from build123d import *

# Parameters (mm, degrees)
SKETCH1_W           = 94
SKETCH1_H           = 90
BOSS_EXTRUDE1_DEPTH = 12
SKETCH2_R           = 4
CUT_EXTRUDE1_DEPTH  = 67.166456759
SKETCH3_R           = 1.6
CUT_EXTRUDE2_DEPTH  = 67.166456759


with BuildPart() as part:
    # Sketch1 → Boss-Extrude1 (new body)
    with BuildSketch(Plane(origin=(0, 0, 0), x_dir=(0, 0, -1), z_dir=(1, 0, 0))):
        Rectangle(SKETCH1_W, SKETCH1_H)
    extrude(amount=BOSS_EXTRUDE1_DEPTH)

    # Sketch2 → Cut-Extrude1 (cut, through all)
    with BuildSketch(Plane(origin=(12, 0, 0), x_dir=(0, 0, -1), z_dir=(1, 0, 0))):
        Circle(SKETCH2_R)
    extrude(amount=-CUT_EXTRUDE1_DEPTH, mode=Mode.SUBTRACT)

    # Sketch3 → Cut-Extrude2 (cut, through all)
    with BuildSketch(Plane.ZY):
        with Locations((0, -20)):
            Circle(SKETCH3_R)
    extrude(amount=-CUT_EXTRUDE2_DEPTH, mode=Mode.SUBTRACT)


solid = part.part
Geometry: final body of the model. Coordinates: model frame, mm. Coordinates: 2 decimals unless noted, no trailing zeros. Loops run counter-clockwise (first coordinate to the right, second up) from the corner with the lowest first, then second, coordinate; pieces in that order, holes last. Notation, with made-up numbers: (41.25, 71) - (75.25, 71) arc R5 ccw to (75.25, 77) - close; hole circle Ø1 at (25.5, 71). An arc over 180 degrees is marked (long way). Put each result on its own line as item: value. Start each with the question number.
Q1. Line query: line 1 (Y direction, x = 4.5, z = 0). Output: solid intervals per line, ascending.
Q2. Cut plane A-A, the plane y = 0. Return loops of the section in (x, z), and give its area (3 significant figures).
Q3. Cut plane C-C, the plane y = -20. Return loops of the section in (x, z).
Q4. Cut plane B-B, the plane z = 0. Return loops of the section in (x, y).
Q5. Pull-direction query (Y, two-part tool) for faces 1 (the cylindrical face through (6.084, -3.905, 0.867)), 2 (the flat face through (6, 45, 1)), 3 (the flat face through (0, 11, 1)), 4 (the flat face through (6, -45, 1)); classes: released by +Y, released by -Y, zero draft, split by the parting line, or undercut.
Filled sheet:
1. line 1: -45 to -21.6, -18.4 to -4, 4 to 45
2. outline: (0, -47) - (12, -47) - (12, -4) - (0, -4) - close; (0, 4) - (12, 4) - (12, 47) - (0, 47) - close
2. area: 1,030 mm²
3. outline: (0, -47) - (12, -47) - (12, -1.6) - (0, -1.6) - close; (0, 1.6) - (12, 1.6) - (12, 47) - (0, 47) - close
4. outline: (0, -45) - (12, -45) - (12, -21.6) - (0, -21.6) - close; (0, -18.4) - (12, -18.4) - (12, -4) - (0, -4) - close; (0, 4) - (12, 4) - (12, 45) - (0, 45) - close
5. face 1: undercut
5. face 2: released by +Y
5. face 3: zero draft
5. face 4: released by -Y
